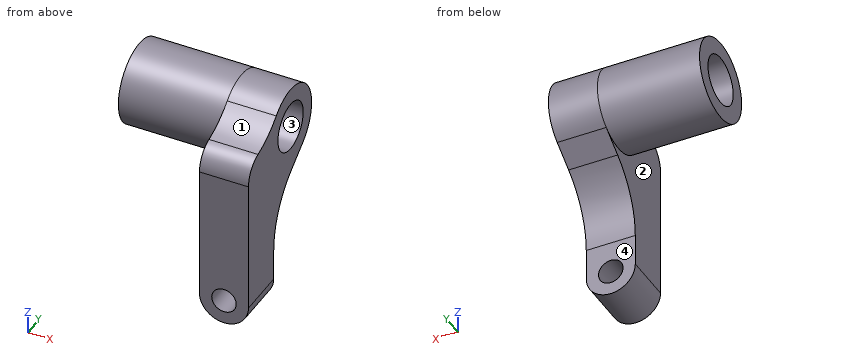
from build123d import *

# Parameters (mm, degrees)
BOSS_EXTRU_1_DEPTH      = 6
CONG_3_R                = 10
BOSS_EXTRU_2_START      = 12.5
ESQUISSE2_R             = 5
BOSS_EXTRU_2_DEPTH      = 12.5
ESQUISSE3_R             = 3
ENL_V_MAT_EXTRU_1_DEPTH = 27.424420523
BOSS_EXTRU_3_DEPTH      = 6
CONG_5_R                = 10
ESQUISSE5_R             = 1.5
ENL_V_MAT_EXTRU_2_DEPTH = 27.043233286
CONG_7_R                = 3


with BuildPart() as part:
    # Esquisse1 → Boss.-Extru.1 (new body)
    with BuildSketch(Plane(origin=(0, 0, 0), x_dir=(0, 0, -1), z_dir=(1, 0, 0))):
        with BuildLine():
            Line((-1, -4.898979486), (-1, -10))
            Line((-1, -10), (16, -10))
            Line((16, -10), (14, -4))
            Line((14, -4), (9, -4))
            Line((9, -4), (4.06913018, 2.905542906))
            ThreePointArc((4.06913018, 2.905542906), (-4.193153044, 2.723502808), (-1, -4.898979486))
        make_face()
    extrude(amount=BOSS_EXTRU_1_DEPTH)

    # Congé3
    # the kernel refuses this fillet: 10 mm, written as the material it adds along each edge
    with BuildSketch(Plane(origin=(0, -4.898979486, 1), x_dir=(0, -1, 0), z_dir=(1, 0, 0))) as cong_3_piece_1:
        with BuildLine():
            CenterArc((5.301220936, -9.997995789), CONG_3_R, 91.147140557, 41.697546603)
            Line((-1.498912679, -2.665998596), (-1.634915351, -2.519358652))
            ThreePointArc((-1.634915351, -2.519358652), (-0.714939835, -1.35240562), (-0.195959179, 0.04))
            Line((-0.195959179, 0.04), (0, 0.2))
            ThreePointArc((0, 0.2), (2.550510257, 0.2), (5.097016506, 0.199959916))
            Line((5.097016506, 0.199959916), (5.101020514, 0))
        make_face()
    extrude(amount=6)

    # Esquisse2 → Boss.-Extru.2 (add)
    with BuildSketch(Plane.ZY.offset(BOSS_EXTRU_2_START)):
        Circle(ESQUISSE2_R)
    extrude(amount=-BOSS_EXTRU_2_DEPTH)

    # Esquisse3 → Enlèv. mat.-Extru.1 (cut, through all)
    with BuildSketch(Plane(origin=(6, 0, 0), x_dir=(0, 0, -1), z_dir=(1, 0, 0))):
        Circle(ESQUISSE3_R)
    extrude(amount=-ENL_V_MAT_EXTRU_1_DEPTH, mode=Mode.SUBTRACT)

    # Esquisse4 → Boss.-Extru.3 (add)
    with BuildSketch(Plane.XZ.offset(10)):
        with BuildLine():
            Line((6, -11), (0, -11))
            Line((0, -11), (0, -18))
            ThreePointArc((0, -18), (3, -21), (6, -18))
            Line((6, -18), (6, -11))
        make_face()
    extrude(amount=-BOSS_EXTRU_3_DEPTH)

    # Congé5
    # the kernel refuses this fillet: 10 mm, written as the material it adds along each edge
    with BuildSketch(Plane(origin=(0, -4, -9), x_dir=(0, 0.813826036051075, 0.5811085811149191), z_dir=(1, 0, 0))) as cong_5_piece_1:
        with BuildLine():
            CenterArc((CONG_5_R * 0.514718625761, -CONG_5_R), CONG_5_R, 90, 54.471447841)
            Line((-CONG_5_R * 0.29910741029, -CONG_5_R * 0.418891418885), (0, 0))
            Line((0, 0), (CONG_5_R * 0.514718625761, 0))
        make_face()
    extrude(amount=6)

    # Esquisse5 → Enlèv. mat.-Extru.2 (cut, through all)
    with BuildSketch(Plane(origin=(0, -4, 0), x_dir=(1, 0, 0), z_dir=(0, 1, 0))):
        with Locations(Location((3, 18, 0), (0, 0, 270))):
            Circle(ESQUISSE5_R)
    extrude(amount=-ENL_V_MAT_EXTRU_2_DEPTH, mode=Mode.SUBTRACT)

    # Congé7
    cong_7_edges = [part.edges().sort_by_distance(p)[0] for p in [
        (3, -10, 1),
    ]]
    fillet(cong_7_edges, radius=CONG_7_R)


solid = part.part
Work out the finished part from the listing and answer in its coordinate system (mm). Face numbers are marked on the shaded views. Give positions to 0.01 mm unless a question says otherwise; leave off trailing zeros. Order: outer loops, then holes, each group sorted by start corner. A loop starts at its lowest first (then second) coordinate and runs counter-clockwise, first axis right, second up. Notation, with made-up numbers: M 81,-4 L 87,-4 A20 cw 87,30 Z; hole C 5.25,-25.5 d5. An arc over 180 degrees is marked long. Return JSON: item names as keys, results as strings.
Q1. Find section D-D, the plane x = -3. Write down the section's boundary in (y, z), and give its area (3 significant figures).
Answer below:
{"outline": "C 0,0 d10; hole C 0,0 d6", "area": "50.3 mm^2"}
Q2. Each of these flat-tipped pins is pushed along its axis until it touches: pin 1 (1.8 mm diameter, centred on x = 4, z = -18, fed in from +Y); pin 2 (2 mm diameter, centred on x = -9, z = -1.5, fed in from +Y); pin 3 (3 mm diameter, centred on x = -7.5, y = -3, fed in from +Z). Where does it stop, or does it pass through?
Answer below:
{"pin 1": "stops at y = -4", "pin 2": "stops at y = 4.97", "pin 3": "stops at z = 4.77"}
Q3. Find section C-C, the plane y = -7. Write down the section's boundary in (x, z), and give its area (3 significant figures).
Answer below:
{"outline": "M 0,-18 A3 ccw 6,-18 L 6,1.52 L 0,1.52 Z; hole C 3,-18 d3", "area": "124 mm^2"}
Q4. The mould has two halves that part along Y. Classify the marked faces 1, 2, 3 and 4: pulls with the +Y half, pulls with the -Y half, needs draft (parallel to the pull), parting line crosses it, or undercut.
Answer below:
{"face 1": "pulls with the -Y half", "face 2": "needs draft", "face 3": "undercut", "face 4": "pulls with the +Y half"}
Q5. Find the intervals of material crossed by line 1 along X through (y, z) = (-8.3, -18); line 2 along Y through (x, z) = (-5, 0); line 3 along X through (y, z) = (-6.5, 0.25), in increasing order. Write a range as [from, to].
Answer below:
{"line 1": "x = [0, 1.5], [4.5, 6]", "line 2": "y = [-5, -3], [3, 5]", "line 3": "x = [0, 6]"}
Q6. Find section B-B, the plane z = 0. Write down the section's boundary in (x, y).
Answer below:
{"outline": "M -12.5,-5 L 0,-5 L 0,-9.54 L 6,-9.54 L 6,-3 L -12.5,-3 Z; M -12.5,3 L 6,3 L 6,5 L -12.5,5 Z"}
